Autodesk Inventor part; units mm, degrees
ref_plane "YZ Plane" through (0, 0, 0) normal (1, 0, 0) x (0, 1, 0)
ref_plane "XZ Plane" through (0, 0, 0) normal (0, 1, 0) x (-1, 0, 0)
ref_plane "XY Plane" through (0, 0, 0) normal (0, 0, 1) x (1, 0, 0)
sketch "スケッチ1" plane through (0, 0, 0) normal (0, 0, 1) x (1, 0, 0)
  circle A0 centre (0, 0) radius 3
  circle A1 centre (0, 0) radius 1.5
  dimension "d0" = 6
  dimension "d1" = 3
extrude "押し出し1" add sketch "スケッチ1" along normal blind 21
fillet "フィレット1" radius 0.3 2 edges at (-3, 0, 21) (-3, 0, 0)
thread "ねじ1"
extrude "押し出し2" add sketch "スケッチ1" along normal blind 15 contours A1
extrude "押し出し3" cut sketch "スケッチ1" along normal blind 6 contours A1
thread "ねじ2"
properties part number "スペーサーM3L21黄銅" material "アルミニウム 2014-T4"
Design review of the part built by this model. Coordinates are the model's own, in mm. A direction names the side the tool comes from. Coordinates: 2 decimals unless noted, no trailing zeros. Order: outer loops, then holes, each group sorted by start corner. A loop starts at its lowest first (then second) coordinate and runs counter-clockwise, first axis right, second up. Notation, with made-up numbers: (29.5, -40) - (87.5, -40) arc R19 ccw to (87.5, -14) - close; hole circle Ø7 at (84.5, 37.5). An arc over 180 degrees is marked (long way). Answer in a Markdown table with one row per item.
(1) Clearance check with flat-ended pins moving along their axes: pin 1 (0.9 mm diameter, centred on x = -0.5, y = 0.5, fed in from -Z); pin 2 (1.5 mm diameter, centred on y = -1, z = 6.5, fed in from +X); pin 3 (1.5 mm diameter, centred on y = 1, z = 18, fed in from -X). State where each tip first meets the part, or that it passes through.
Checked values:
| item | result |
|---|---|
| pin 1 | z = 6 |
| pin 2 | x = 2.99 |
| pin 3 | x = -2.99 |
(2) For faces 1 (the cylindrical face through (-1.5, -0.07, 2.96)), 2 (the cylindrical face through (-1.5, -0.07, 17.96)), 3 (the flat face through (1.2, -1.2, 0)), list the 3-axis set-ups (+Z, -Z, +X, -X, +Y, -Y) from which the entire face can be reached by the end or side of a thin tool; tool diameter is ignored.
Checked values:
| item | result |
|---|---|
| face 1 | -Z |
| face 2 | +Z |
| face 3 | -Z, +X, -X, +Y, -Y |
(3) Consider section A-A on x = 0. State the section outline as (y, z) points.
Checked values:
| item | result |
|---|---|
| outline | (-3, 0.3) arc R0.3 ccw to (-2.7, 0) - (-1.5, 0) - (-1.5, 6) - (1.5, 6) - (1.5, 0) - (2.7, 0) arc R0.3 ccw to (3, 0.3) - (3, 20.7) arc R0.3 ccw to (2.7, 21) - (1.5, 21) - (1.5, 15) - (-1.5, 15) - (-1.5, 21) - (-2.7, 21) arc R0.3 ccw to (-3, 20.7) - close |
(4) Wall thickness on line 1 along Y through (x, z) = (0, 19.7); line 2 along Z through (x, y) = (1.25, -0.75); line 3 along Y through (x, z) = (1, 16): over which ranges is each line inside the solid? List them lowest first. Write a range as from..to.
Checked values:
| item | result |
|---|---|
| line 1 | -3..-1.5, 1.5..3 |
| line 2 | 6..15 |
| line 3 | -2.83..-1.12, 1.12..2.83 |
(5) Consider section D-D on z = 16. State the section outline as (x, y) points.
Checked values:
| item | result |
|---|---|
| outline | circle Ø6 at (0, 0); hole circle Ø3 at (0, 0) |
(6) The part is to be moulded in two halves that separate along Y. For faces 4 (the cylindrical face through (-3, 0, 10)), 5 (the flat face through (0, 0, 15)), 6 (the flat face through (1.2, -1.2, 21)), say which applies: released by +Y, released by -Y, zero draft, split by the parting line, or undercut.
Checked values:
| item | result |
|---|---|
| face 4 | split by the parting line |
| face 5 | undercut |
| face 6 | zero draft |
(7) Consider section C-C on z = 9. State the section outline as (x, y) points, plus the area to 3 significant figures.
Checked values:
| item | result |
|---|---|
| outline | circle Ø6 at (0, 0) |
| area | 28.3 mm^2 |
